```python
from build123d import *

# Parameters (mm, degrees)
SKETCH_1_R      = 6
EXTRUDE_1_DEPTH = 350
SKETCH_2_W      = 4
SKETCH_2_H      = 9.160592614
EXTRUDE_2_DEPTH = 23.51


with BuildPart() as part:
    # 草图1 → 凸台-拉伸1 (new body)
    with BuildSketch(Plane.XY):
        Circle(SKETCH_1_R)
    extrude(amount=EXTRUDE_1_DEPTH)

    # 草图2 → 凸台-拉伸2 (add)
    with BuildSketch(Plane.XY.offset(350)):
        with Locations((0, 3.419703693)):
            Rectangle(SKETCH_2_W, SKETCH_2_H)
    extrude(amount=-EXTRUDE_2_DEPTH)


solid = part.part
```
The model under review builds one solid part; all positions refer to its coordinate system, in mm. Give positions to 0.01 mm unless a question says otherwise; leave off trailing zeros. Write each loop counter-clockwise with the first axis right and the second up, starting at its lowest first coordinate (ties: lowest second). Pieces come first, ordered by that corner, then holes. Notation, with made-up numbers: (53.25, -6.5) - (111.25, -6.5) arc R4 ccw to (111.25, 0.5) - close; hole circle Ø3 at (20, 70). An arc over 180 degrees is marked (long way). Answer in a Markdown table with one row per item. Add a question column.
1. We need section A-A on x = 0. Write out the cut boundary in (y, z).
2. Wall thickness on line 1 along X through (y, z) = (-0.5, 199); line 2 along Z through (x, y) = (-1.25, 7.25); line 3 along Y through (x, z) = (-0.25, 326): over which ranges is each line inside the solid? List them lowest first. Write a range as [from, to].
3. We need section B-B on z = 94. Write out the cut boundary in (x, y), then the cut area to 3 significant figures.
4. We need section C-C on y = 3.25. Write out the cut boundary in (x, z).
5. Insertion check: P1, Ø1, axis at y = -4.5, z = 100, coming from the +X side; P2, Ø2, axis at x = -4, z = 115.5, coming from the -Y side; P3, Ø1.9, axis at y = 6.5, z = 335, coming from the -X side. Each pin has a flat end and moves straight along its axis. Give the tip position at first contact, or say it passes through.
Ans:
| question | item | result |
|---|---|---|
| 1 | outline | (-6, 0) - (6, 0) - (6, 326.49) - (8, 326.49) - (8, 350) - (-6, 350) - close |
| 2 | line 1 | x = [-5.98, 5.98] |
| 2 | line 2 | z = [326.49, 350] |
| 2 | line 3 | y = [-5.99, 5.99] |
| 3 | outline | circle Ø12 at (0, 0) |
| 3 | area | 113 mm^2 |
| 4 | outline | (-5.04, 0) - (5.04, 0) - (5.04, 350) - (-5.04, 350) - close |
| 5 | P1 | stops at x = 4.47 |
| 5 | P2 | stops at y = -5.2 |
| 5 | P3 | stops at x = -2.28 |
